Here's how the part is built. I have some questions about the finished solid (model axes, mm). A direction names the side the tool comes from. Coordinates: 2 decimals unless noted, no trailing zeros. Write each loop counter-clockwise with the first axis right and the second up, starting at its lowest first coordinate (ties: lowest second). Pieces come first, ordered by that corner, then holes.
(1) Imagine slicing it at C-C, the plane z = -74. List the corners of the cut face in (x, y) for me, plus the area to 3 significant figures.
(2) Thinking about a two-plate mould opening in Z: for faces 1 (the flat face through (1, -10, 29)), 2 (the cylindrical face through (-35.437, 11.189, 23.084)), 3 (the flat face through (1, -10, -17)), which applies, released by +Z, released by -Z, zero draft, split by the parting line, or undercut?
(3) Which directions (+Z, -Z, +X, -X, +Y, -Y) give clear straight access to the entire face, cutting with the end or side of a thin tool? Please do faces 4 (the flat face through (-17, -28, -61)), 5 (the flat face through (0, -19, -54)), 6 (the flat face through (0, 6, -23)).
(4) Imagine slicing it at B-B, the plane x = 0. List the corners of the cut face in (y, z) for me.
(5) Imagine slicing it at A-A, the plane y = -12. List the corners of the cut face in (x, z) for me.
(6) Please list where these lines run through material, in increasing order: probe 1 along Y at (x, z) = (14, 19.5); probe 2 along Z at (x, y) = (-21.5, -6.5); probe 3 along Z at (x, y) = (0, -32.25).
(7) For pin 1 Ø3 at (y, z) = (5.5, 16.5) entering from +X; pin 2 Ø10 at (x, z) = (3.5, 7) entering from +Y; pin 3 Ø2 at (x, y) = (-31, -27) entering from -Z, each with a flat end and sliding along its axis, tell me the tip position at first contact or that it passes through.
(8) Imagine slicing it at D-D, the plane z = 14.5. List the corners of the cut face in (x, y) for me.
```python
from build123d import *

# Parameters (mm, degrees)
EXTRUDE_2_DEPTH          = 29
SKETCH_3_W               = 34
SKETCH_3_H               = 35
CUT_EXTRUDE_1_DEPTH      = 41
CUT_EXTRUDE_1_DEPTH_BACK = 41
SKETCH_4_R               = 8
EXTRUDE_3_DEPTH          = 17


with BuildPart() as part:
    # 草圖1 → 填料-伸長2 (new body, symmetric)
    with BuildSketch(Plane.XY):
        with BuildLine():
            Line((-24, 16), (24, 16))
            ThreePointArc((24, 16), (35.313708499, 11.313708499), (40, 0))
            Line((40, 0), (40, -36))
            Line((40, -36), (-40, -36))
            Line((-40, -36), (-40, 0))
            ThreePointArc((-40, 0), (-35.313708499, 11.313708499), (-24, 16))
        make_face()
        with BuildLine():
            Line((-24, 6), (24, 6))
            ThreePointArc((24, 6), (30, 0), (24, -6))
            Line((24, -6), (-24, -6))
            ThreePointArc((-24, -6), (-30, 0), (-24, 6))
        make_face(mode=Mode.SUBTRACT)
    extrude(amount=EXTRUDE_2_DEPTH, both=True)

    # 草圖3 → 除料-伸長1 (cut, two sides)
    with BuildSketch(Plane(origin=(0, 0, 0), x_dir=(0, 0, -1), z_dir=(1, 0, 0))) as cut_extrude_1_sk:
        with Locations((0, -1.5)):
            Rectangle(SKETCH_3_W, SKETCH_3_H)
    extrude(amount=CUT_EXTRUDE_1_DEPTH, mode=Mode.SUBTRACT)
    extrude(cut_extrude_1_sk.sketch, amount=-CUT_EXTRUDE_1_DEPTH_BACK, mode=Mode.SUBTRACT)

    # 草圖4 → 填料-伸長3 (add)
    with BuildSketch(Plane.XZ.offset(36)):
        with BuildLine():
            Line((-17, -77), (-17, -45))
            ThreePointArc((-17, -45), (-21.686291501, -33.686291501), (-33, -29))
            Line((-33, -29), (33, -29))
            ThreePointArc((33, -29), (21.686291501, -33.686291501), (17, -45))
            Line((17, -45), (17, -77))
            ThreePointArc((17, -77), (0, -94), (-17, -77))
        make_face()
        with Locations((0, -77)):
            Circle(SKETCH_4_R, mode=Mode.SUBTRACT)
    extrude(amount=-EXTRUDE_3_DEPTH)


solid = part.part
```
Recorded:
1. outline: (-17, -36) - (-7.42, -36) - (-7.42, -19) - (-17, -19) - close; (7.42, -36) - (17, -36) - (17, -19) - (7.42, -19) - close
1. area: 326 mm2
2. face 1: released by +Z
2. face 2: zero draft
2. face 3: undercut
3. face 4: -Z, -X, +Y, -Y
3. face 5: -Z, +X, -X, +Y
3. face 6: +Z, -Z
4. outline: (-36, -94) - (-19, -94) - (-19, -85) - (-36, -85) - close; (-36, -69) - (-19, -69) - (-19, -29) - (-6, -29) - (-6, -17) - (-19, -17) - (-19, 17) - (-6, 17) - (-6, 29) - (-36, 29) - close; (6, -29) - (16, -29) - (16, -17) - (6, -17) - close; (6, 17) - (16, 17) - (16, 29) - (6, 29) - close
5. outline: (-40, -29) - (40, -29) - (40, -17) - (-40, -17) - close; (-40, 17) - (40, 17) - (40, 29) - (-40, 29) - close
6. probe 1: y = -36 to -6, 6 to 16
6. probe 2: z = -29 to -17, 17 to 29
6. probe 3: z = -94 to -85, -69 to 29
7. pin 1: stops at x = 39.47
7. pin 2: stops at y = -19
7. pin 3: stops at z = -29.28
8. outline: (-40, -36) - (40, -36) - (40, -19) - (-40, -19) - close
